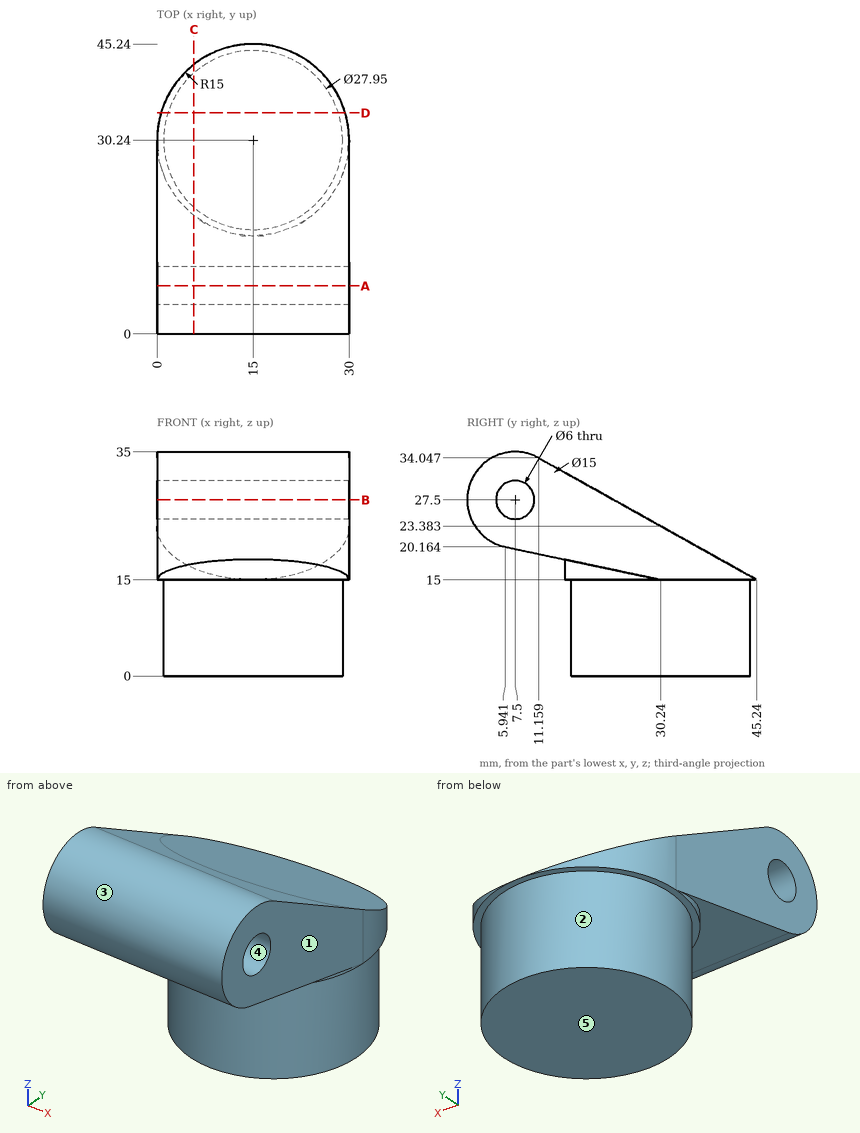
Job drawing, mm, ordinate dimensions from the low corner. One solid piece. A direction names the side the tool comes from. Give positions to 0.01 mm unless a question says otherwise; leave off trailing zeros. Write each loop counter-clockwise with the first axis right and the second up, starting at its lowest first coordinate (ties: lowest second). Pieces come first, ordered by that corner, then holes. Notation, with made-up numbers: (33, 2) - (89, 2) arc R17 cw to (89, 7) - close; hole circle Ø2 at (24.25, 28.25). An arc over 180 degrees is marked (long way). Answer as CSV lines item,"result".
1. Two-plate mould, pull along Y, no slides. Class the marked faces 3, 4 and 5: +Y half, -Y half, draft (parallel to the pull), parting line (faces both ways), or undercut.
Responses:
face 3,"parting line"
face 4,"undercut"
face 5,"draft"
2. Band-saw the part on D-D (y = 34.5). Write the cut outline in (x, z).
Responses:
outline,"(0.62, 15) - (1.69, 15) - (1.69, 0) - (28.31, 0) - (28.31, 15) - (29.38, 15) - (29.38, 21) - (0.62, 21) - close"
3. 3-axis set-ups, long thin cutter, end or side, ignore diameter. For the marked faces 1 and 2: which of +Z, -Z, +X, -X, +Y, -Y reach the whole face in a straight line?
Responses:
face 1,"+Z, -Z, +X, +Y, -Y"
face 2,"-Z"
4. Pin check, flat tips, straight feed: pin 1 (3 mm diameter, centred on x = 7, z = 25.5, fed in from -Y); pin 2 (4 mm diameter, centred on y = 39, z = 19, fed in from +X); pin 3 (3 mm diameter, centred on x = 25.5, y = 12, fed in from +Z). Stop position of each tip, or through.
Responses:
pin 1,"stops at y = 0.02"
pin 2,"stops at x = 28.39"
pin 3,"stops at z = 34.37"
5. Band-saw the part on B-B (z = 27.5). Write the cut outline in (x, y), and give its area (3 significant figures).
Responses:
outline,"(0, 0) - (30, 0) - (30, 4.5) - (0, 4.5) - close; (0, 10.5) - (30, 10.5) - (30, 22.87) - (0, 22.87) - close"
area,"506 mm2"
6. Drill centre lines: L1, parallel to Y at x = 23.75, z = 27.5 (1 decimal); L2, parallel to Z at x = 23, y = 5; L3, parallel to X at y = 19, z = 2 (1 decimal). Where is each one in solid material? Low to high. Write a range as [from, to].
Responses:
L1,"y = [0, 4.5], [10.5, 22.9]"
L2,"z = [20.43, 25.84], [29.16, 34.57]"
L3,"x = [6.7, 23.3]"
7. Band-saw the part on C-C (x = 5.75). Write the cut outline in (y, z), and give its area (3 significant figures).
Responses:
outline,"(5.94, 20.16) - (18.43, 17.51) - (18.43, 15) - (19.76, 15) - (19.76, 0) - (40.72, 0) - (40.72, 15) - (42.05, 15) - (42.05, 16.78) - (11.16, 34.05) arc R7.5 ccw (long way) to start; hole circle Ø6 at (7.5, 27.5)"
area,"728 mm2"
8. Band-saw the part on A-A (y = 7.5). Write the cut outline in (x, z), and give its area (3 significant figures).
Responses:
outline,"(0, 19.83) - (30, 19.83) - (30, 24.5) - (0, 24.5) - close; (0, 30.5) - (30, 30.5) - (30, 35) - (0, 35) - close"
area,"275 mm2"
